Could you check a few things on this model? Use its own coordinates, in mm. Face numbers are marked on the shaded views. A direction names the side the tool comes from. Round coordinates to 2 decimals unless told otherwise and drop trailing zeros. Loops run counter-clockwise (first coordinate to the right, second up) from the corner with the lowest first, then second, coordinate; pieces in that order, holes last. Notation, with made-up numbers: (80, 75) -> (85, 75) arc R29 ccw to (85, 100) -> close; hole circle Ø11 at (45.5, 14). An arc over 180 degrees is marked (long way). Write each question's results on one line, items separated by ' | '.
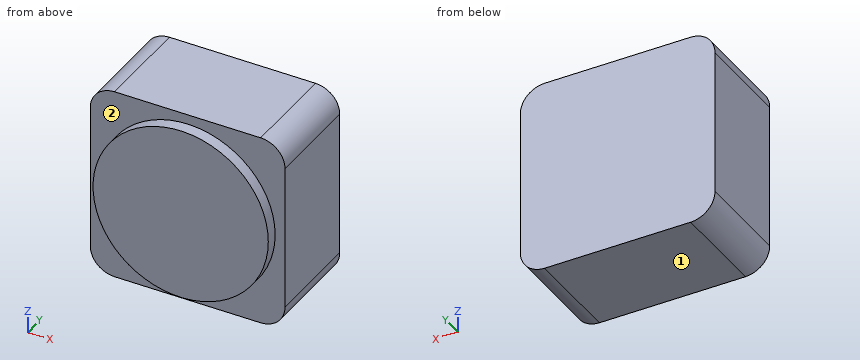
from build123d import *

# Parameters (mm, degrees)
F0_W     = 40
F0_H     = 40
F1_DEPTH = 20
F2_R     = 5
F3_R     = 18
F4_DEPTH = 2.5


with BuildPart() as f1:
    # F0 (on Front) → F1 (new body)
    with BuildSketch(Plane.XZ):
        with Locations((20, 20)):
            Rectangle(F0_W, F0_H)
    extrude(amount=F1_DEPTH)

    # F2
    f2_edges = [f1.edges().sort_by_distance(p)[0] for p in [
        (0, -10, 40),
        (40, -10, 40),
        (0, -10, 0),
        (40, -10, 0),
    ]]
    fillet(f2_edges, radius=F2_R)

    # F3 (on face) → F4 (join)
    with BuildSketch(Plane.XZ.offset(20)):
        with Locations((19.97735, 20)):
            Circle(F3_R)
    extrude(amount=F4_DEPTH)


solid = f1.part
1) I want a section at A-A, the plane x = 31. Write out the boundary of the cut face in (y, z), plus the area to 3 significant figures.
Model answer:
outline: (-22.5, 5.77) -> (-20, 5.77) -> (-20, 0) -> (0, 0) -> (0, 40) -> (-20, 40) -> (-20, 34.23) -> (-22.5, 34.23) -> close | area: 871 mm2
2) I want a section at C-C, the plane y = -20.5. Write out the boundary of the cut face in (x, z).
Model answer:
outline: circle Ø36 at (19.98, 20)
3) I'm going to push a flat-ended pin straight in: pin 1 (3 mm diameter, centred on x = 18.5, z = 17.5, fed in from +Y). Where does the tip first touch, or does it pass through?
Model answer:
pin 1: stops at y = 0
4) I want a section at B-B, the plane z = 31.5. Write out the boundary of the cut face in (x, y).
Model answer:
outline: (0, -20) -> (6.13, -20) -> (6.13, -22.5) -> (33.82, -22.5) -> (33.82, -20) -> (40, -20) -> (40, 0) -> (0, 0) -> close
5) I need wall thicknesses on line 1 (Y direction, x = 8, z = 37); line 2 (Z direction, x = 3, y = -2.5); line 3 (X direction, y = -19.5, z = 38.5). Which ranges of each line are inside material? Lowest first, please.
Model answer:
line 1: y = -20 to 0 | line 2: z = 0.42 to 39.58 | line 3: x = 1.43 to 38.57
6) For the marked faces 1 and 2, which set-ups out of +Z, -Z, +X, -X, +Y, -Y let a thin tool reach every point of the face, with its end or its side?
Model answer:
face 1: -Z, +X, -X, +Y, -Y | face 2: -Y
